The listing builds one solid part. Answer for the finished solid, in the listing's coordinates (mm). Face numbers are marked on the shaded views. A direction names the side the tool comes from. Give positions to 0.01 mm unless a question says otherwise; leave off trailing zeros. Loops run counter-clockwise (first coordinate to the right, second up) from the corner with the lowest first, then second, coordinate; pieces in that order, holes last. Notation, with made-up numbers: (-9.5, 87) - (-2.5, 87) arc R21 cw to (-2.5, 111) - close; hole circle Ø2 at (54.5, 62). An arc over 180 degrees is marked (long way). Answer in a Markdown table with one row per item. Add a question column.
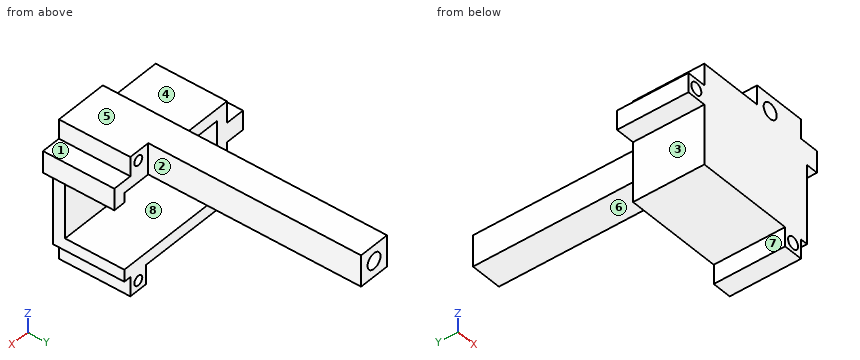
```python
from build123d import *

# Parameters (mm, degrees)
BOSS_EXTRUDE1_DEPTH  = 24.5
SKETCH2_W            = 103
SKETCH2_H            = 41.85
BOSS_EXTRUDE2_DEPTH  = 5
SKETCH3_W            = 46.5
SKETCH3_H            = 27.85
CUT_EXTRUDE1_DEPTH   = 26
SKETCH7_W            = 8
SKETCH7_H            = 3
BOSS_EXTRUDE3_DEPTH  = 8
SKETCH8_R            = 2.5
CUT_EXTRUDE2_DEPTH   = 8
SKETCH9_W            = 8
SKETCH9_H            = 3
BOSS_EXTRUDE4_DEPTH  = 8
SKETCH10_R           = 2.5
CUT_EXTRUDE3_DEPTH   = 8
SKETCH12_W           = 11.5
SKETCH12_H           = 5
CUT_EXTRUDE4_DEPTH   = 8
SKETCH14_W           = 8
SKETCH14_H           = 3
BOSS_EXTRUDE5_DEPTH  = 8
SKETCH15_R           = 2.5
CUT_EXTRUDE5_DEPTH   = 8
SKETCH16_W           = 8
SKETCH16_H           = 29.5
BOSS_EXTRUDE6_DEPTH  = 8
SKETCH17_W           = 14
SKETCH17_H           = 29.5
BOSS_EXTRUDE7_DEPTH  = 8
SKETCH18_R           = 2
CUT_EXTRUDE6_DEPTH   = 10
SKETCH19_W           = 8
SKETCH19_H           = 29.5
BOSS_EXTRUDE8_DEPTH  = 8
SKETCH20_W           = 13
SKETCH20_H           = 13
BOSS_EXTRUDE9_DEPTH  = 88
CUT_EXTRUDE8_DEPTH   = 48
SKETCH23_R           = 2.5
CUT_EXTRUDE9_DEPTH   = 10
SKETCH26_R           = 3.25
CUT_EXTRUDE11_DEPTH  = 117.5
SKETCH25_W           = 8
SKETCH25_H           = 3
CUT_EXTRUDE10_DEPTH  = 8
SKETCH27_W           = 8
SKETCH27_H           = 29.5
BOSS_EXTRUDE11_DEPTH = 8
SKETCH28_R           = 2.5
CUT_EXTRUDE12_DEPTH  = 15


with BuildPart() as part:
    # Sketch1 → Boss-Extrude1 (new body)
    with BuildSketch(Plane(origin=(0, 0, 0), x_dir=(1, 0, 0), z_dir=(0, 1, 0))):
        Polygon((0, 0), (51.5, 0), (51.5, -5), (5, -5), (5, -36.85), (51.5, -36.85), (51.5, -32.85), (56.5, -32.85), (56.5, -41.85), (0, -41.85), align=None)
    extrude(amount=BOSS_EXTRUDE1_DEPTH)

    # Sketch2 → Boss-Extrude2 (add)
    with BuildSketch(Plane.XZ):
        with Locations((51.5, 20.925)):
            Rectangle(SKETCH2_W, SKETCH2_H)
    extrude(amount=BOSS_EXTRUDE2_DEPTH)

    # Sketch3 → Cut-Extrude1 (cut)
    with BuildSketch(Plane(origin=(0, 0, 0), x_dir=(1, 0, 0), z_dir=(0, 1, 0))):
        with Locations((74.75, -18.925)):
            Rectangle(SKETCH3_W, SKETCH3_H)
    extrude(amount=-CUT_EXTRUDE1_DEPTH, mode=Mode.SUBTRACT)

    # Sketch7 → Boss-Extrude3 (add)
    with BuildSketch(Plane.XY.offset(41.85)):
        with Locations((4, -3.5)):
            Rectangle(SKETCH7_W, SKETCH7_H)
    extrude(amount=BOSS_EXTRUDE3_DEPTH)

    # Sketch8 → Cut-Extrude2 (cut)
    with BuildSketch(Plane(origin=(0, -2, 0), x_dir=(1, 0, 0), z_dir=(0, 1, 0))):
        with Locations(Location((4, -45.85, 0), (0, 0, 270))):
            Circle(SKETCH8_R)
    extrude(amount=-CUT_EXTRUDE2_DEPTH, mode=Mode.SUBTRACT)

    # Sketch9 → Boss-Extrude4 (add)
    with BuildSketch(Plane(origin=(0, 0, 0), x_dir=(-1, 0, 0), z_dir=(0, 0, -1))):
        with Locations((-99, -3.5)):
            Rectangle(SKETCH9_W, SKETCH9_H)
    extrude(amount=BOSS_EXTRUDE4_DEPTH)

    # Sketch10 → Cut-Extrude3 (cut)
    with BuildSketch(Plane(origin=(0, -2, 0), x_dir=(1, 0, 0), z_dir=(0, 1, 0))):
        with Locations(Location((99, 3.996680608, 0), (0, 0, 270))):
            Circle(SKETCH10_R)
    extrude(amount=-CUT_EXTRUDE3_DEPTH, mode=Mode.SUBTRACT)

    # Sketch12 → Cut-Extrude4 (cut)
    with BuildSketch(Plane(origin=(0, 0, 0), x_dir=(1, 0, 0), z_dir=(0, 1, 0))):
        with Locations((89.25, -2.5)):
            Rectangle(SKETCH12_W, SKETCH12_H)
    extrude(amount=-CUT_EXTRUDE4_DEPTH, mode=Mode.SUBTRACT)

    # Sketch14 → Boss-Extrude5 (add)
    with BuildSketch(Plane(origin=(0, 0, 0), x_dir=(-1, 0, 0), z_dir=(0, 0, -1))):
        with Locations((-79.5, -3.5)):
            Rectangle(SKETCH14_W, SKETCH14_H)
    extrude(amount=BOSS_EXTRUDE5_DEPTH)

    # Sketch15 → Cut-Extrude5 (cut)
    with BuildSketch(Plane(origin=(0, -2, 0), x_dir=(1, 0, 0), z_dir=(0, 1, 0))):
        with Locations(Location((79.5, 4, 0), (0, 0, 270))):
            Circle(SKETCH15_R)
    extrude(amount=-CUT_EXTRUDE5_DEPTH, mode=Mode.SUBTRACT)

    # Sketch16 → Boss-Extrude6 (add)
    with BuildSketch(Plane(origin=(0, 0, 0), x_dir=(-1, 0, 0), z_dir=(0, 0, -1))):
        with Locations((-44.5, 9.75)):
            Rectangle(SKETCH16_W, SKETCH16_H)
    extrude(amount=BOSS_EXTRUDE6_DEPTH)

    # Sketch17 → Boss-Extrude7 (add)
    with BuildSketch(Plane.XY.offset(41.85)):
        with Locations((41.5, 9.75)):
            Rectangle(SKETCH17_W, SKETCH17_H)
    extrude(amount=BOSS_EXTRUDE7_DEPTH)

    # Sketch18 → Cut-Extrude6 (cut)
    with BuildSketch(Plane(origin=(0, 24.5, 0), x_dir=(1, 0, 0), z_dir=(0, 1, 0))):
        with Locations(Location((44.5, 4, 0), (0, 0, 270))):
            Circle(SKETCH18_R)
        with Locations(Location((44.5, -45.85, 0), (0, 0, 270))):
            Circle(SKETCH18_R)
    extrude(amount=-CUT_EXTRUDE6_DEPTH, mode=Mode.SUBTRACT)

    # Sketch19 → Boss-Extrude8 (add)
    with BuildSketch(Plane.ZY.offset(-34.5)):
        with Locations((45.85, 9.75)):
            Rectangle(SKETCH19_W, SKETCH19_H)
    extrude(amount=BOSS_EXTRUDE8_DEPTH)

    # Sketch20 → Boss-Extrude9 (add)
    with BuildSketch(Plane(origin=(0, 24.5, 0), x_dir=(1, 0, 0), z_dir=(0, 1, 0))):
        with Locations((33, -43.35)):
            Rectangle(SKETCH20_W, SKETCH20_H)
    extrude(amount=BOSS_EXTRUDE9_DEPTH)

    # Sketch22 → Cut-Extrude8 (cut)
    with BuildSketch(Plane(origin=(0, 0, 0), x_dir=(1, 0, 0), z_dir=(0, 1, 0))):
        Polygon((103, 0), (103, 8), (51.5, 8), (51.5, -32.85), (56.5, -32.85), (98, -32.85), (98, -5), (95, -5), (95, 0), align=None)
        Polygon((103, -41.85), (103, -32.85), (98, -32.85), (56.5, -32.85), (56.5, -41.85), align=None)
        Polygon((103, -32.85), (103, 0), (95, 0), (95, -5), (98, -5), (98, -32.85), align=None)
    extrude(amount=-CUT_EXTRUDE8_DEPTH, mode=Mode.SUBTRACT)

    # Sketch23 → Cut-Extrude9 (cut)
    with BuildSketch(Plane.XZ.offset(5)):
        with Locations(Location((44.5, -4, 0), (0, 0, 270))):
            Circle(SKETCH23_R)
    extrude(amount=-CUT_EXTRUDE9_DEPTH, mode=Mode.SUBTRACT)

    # Sketch26 → Cut-Extrude11 (cut)
    with BuildSketch(Plane(origin=(0, 112.5, 0), x_dir=(1, 0, 0), z_dir=(0, 1, 0))):
        with Locations(Location((33, -43.35, 0), (0, 0, 270))):
            Circle(SKETCH26_R)
    extrude(amount=-CUT_EXTRUDE11_DEPTH, mode=Mode.SUBTRACT)

    # Sketch25 → Cut-Extrude10 (cut)
    with BuildSketch(Plane.XY.offset(49.85)):
        with Locations((4, -3.5)):
            Rectangle(SKETCH25_W, SKETCH25_H)
    extrude(amount=-CUT_EXTRUDE10_DEPTH, mode=Mode.SUBTRACT)

    # Sketch27 → Boss-Extrude11 (add)
    with BuildSketch(Plane.ZY):
        with Locations((28.85, 9.75)):
            Rectangle(SKETCH27_W, SKETCH27_H)
    extrude(amount=BOSS_EXTRUDE11_DEPTH)

    # Sketch28 → Cut-Extrude12 (cut)
    with BuildSketch(Plane.XZ.offset(5)):
        with Locations(Location((-4, 28.85, 0), (0, 0, 270))):
            Circle(SKETCH28_R)
    extrude(amount=-CUT_EXTRUDE12_DEPTH, mode=Mode.SUBTRACT)


solid = part.part
```
(1) A tool of negligible diameter and unlimited length cuts with its end or side. For the marked faces 1, 2, 3 and 4, from which of +Z, -Z, +X, -X, +Y, -Y can it reach the whole face along a straight path? Write none if from no direction.
(2) A cutting plane is placed at C-C on z = -4. Determine the outline of the cut face in (x, y), plus the area to 3 significant figures.
(3) The mould has two halves that part along Z. Classify the marked faces 5, 6, 7 and 8: pulls with the +Z half, pulls with the -Z half, needs draft (parallel to the pull), parting line crosses it, or undercut.
(4) A cutting plane is placed at D-D on x = 24.5. Determine the outline of the cut face in (y, z).
(5) A cutting plane is placed at B-B on y = 50.5. Determine the outline of the cut face in (x, z), plus the area to 3 significant figures.
(6) Given pin 1 Ø1.2 at (x, z) = (45, -4.5) entering from +Y; pin 2 Ø3 at (y, z) = (42.5, 44) entering from +X; pin 3 Ø15 at (x, y) = (24.5, 6.5) entering from -Z, each flat-ended and moving along its own axis, determine where each tip first touches the part or whether it passes through.
(7) Find the intervals of material crossed by line 1 along X through (y, z) = (-2.5, -4); line 2 along X through (y, z) = (20.75, 45.85); line 3 along X through (y, z) = (22.25, -4), in increasing order. Write a range as [from, to].
(8) A cutting plane is placed at A-A on x = -4. Determine the outline of the cut face in (y, z).
Evaluation:
| question | item | result |
|---|---|---|
| 1 | face 1 | +Z, +X, +Y, -Y |
| 1 | face 2 | +Z, -Z, +X, +Y |
| 1 | face 3 | -Z, -X, +Y, -Y |
| 1 | face 4 | +Z, -X, +Y, -Y |
| 2 | outline | (40.5, -5) - (42, -5) - (42, 5) - (47, 5) - (47, -5) - (48.5, -5) - (48.5, 24.5) - (46.5, 24.5) - (46.5, 14.5) - (42.5, 14.5) - (42.5, 24.5) - (40.5, 24.5) - close |
| 2 | area | 146 mm² |
| 3 | face 5 | pulls with the +Z half |
| 3 | face 6 | undercut |
| 3 | face 7 | needs draft |
| 3 | face 8 | undercut |
| 4 | outline | (-5, 0) - (24.5, 0) - (24.5, 5) - (0, 5) - (0, 36.85) - (24.5, 36.85) - (24.5, 41.85) - (-5, 41.85) - close |
| 5 | outline | (26.5, 36.85) - (39.5, 36.85) - (39.5, 49.85) - (26.5, 49.85) - close; hole circle Ø6.5 at (33, 43.35) |
| 5 | area | 136 mm² |
| 6 | pin 1 | stops at y = 14.5 |
| 6 | pin 2 | stops at x = 39.5 |
| 6 | pin 3 | stops at z = 0 |
| 7 | line 1 | x = [40.5, 42], [47, 48.5] |
| 7 | line 2 | x = [26.5, 30.92], [35.08, 42.5], [46.5, 48.5] |
| 7 | line 3 | x = [40.5, 42.5], [46.5, 48.5] |
| 8 | outline | (-5, 24.85) - (24.5, 24.85) - (24.5, 32.85) - (-5, 32.85) - (-5, 31.35) - (10, 31.35) - (10, 26.35) - (-5, 26.35) - close |
